The figure shows three views and two pictorial views of one solid part (mm, origin at its lowest corner). Answer the questions. Round coordinates to 2 decimals unless told otherwise and drop trailing zeros. Write each loop counter-clockwise with the first axis right and the second up, starting at its lowest first coordinate (ties: lowest second). Pieces come first, ordered by that corner, then holes. Notation, with made-up numbers: M 10,-19.75 L 63,-19.75 A34 ccw 63,12.25 Z; hole C -12,50.5 d11. An arc over 180 degrees is marked long. One line per item, written item: value. Start each with the question number.
Q1. Find section B-B (x = 10.35). Write down the section's boundary in (y, z) (3 decimals), and give its area (3 significant figures).
Q2. Find section A-A (y = 82.55). Write down the section's boundary in (x, z) (3 decimals), and give its area (3 significant figures).
Q3. Consider probe 1 along X at (y, z) = (82.55, 2.7) (3 decimals); probe 2 along Y at (x, z) = (10.35, 2.9) (3 decimals); probe 3 along Y at (x, z) = (7, 2.7). Determine where each line is inside the solid, lowest interval first.
Q4. Given pin 1 Ø1.2 at (y, z) = (1.5, 2.5) entering from -X; pin 2 Ø2 at (x, z) = (33, 2.5) entering from +Y; pin 3 Ø2 at (x, z) = (23.5, 2.5) entering from -Y, each flat-ended and moving along its own axis, determine where each tip first touches the part or whether it passes through.
Q5. Find section D-D (x = 88). Write down the section's boundary in (y, z), and give its area (3 significant figures).
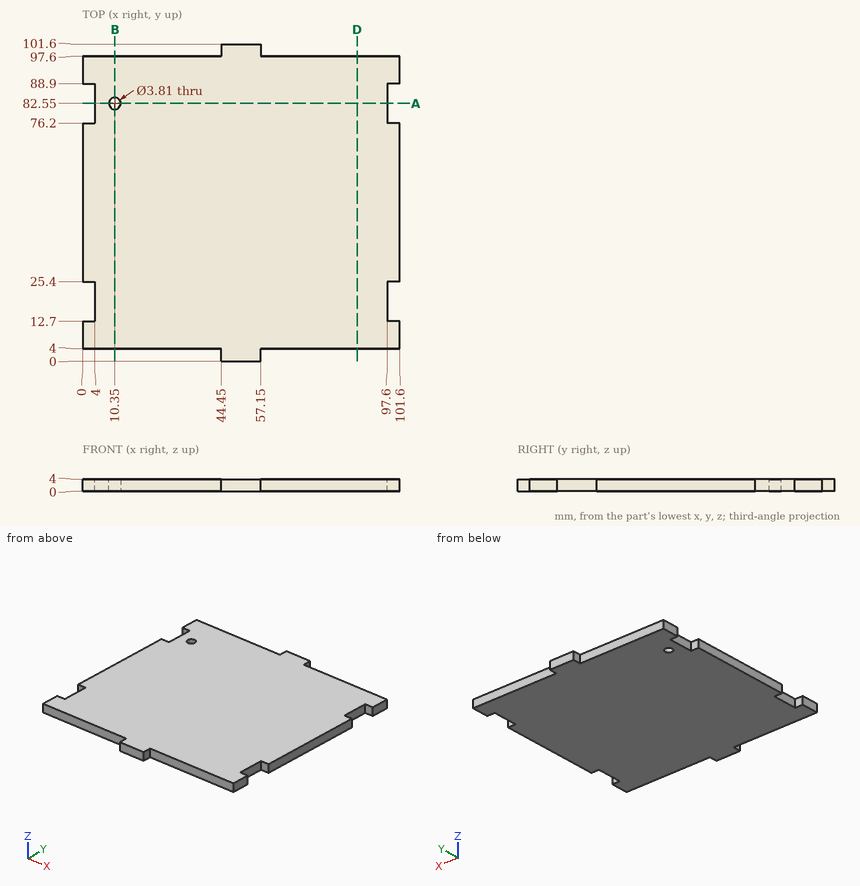
The answers:
1. outline: M 4,0 L 80.645,0 L 80.645,4 L 4,4 Z; M 84.455,0 L 97.6,0 L 97.6,4 L 84.455,4 Z
1. area: 359 mm2
2. outline: M 4,0 L 8.445,0 L 8.445,4 L 4,4 Z; M 12.255,0 L 97.6,0 L 97.6,4 L 12.255,4 Z
2. area: 359 mm2
3. probe 1: 4 to 8.445, 12.255 to 97.6
3. probe 2: 4 to 80.645, 84.455 to 97.6
3. probe 3: 4 to 97.6
4. pin 1: x = 44.45
4. pin 2: y = 97.6
4. pin 3: y = 4
5. outline: M 4,0 L 97.6,0 L 97.6,4 L 4,4 Z
5. area: 374 mm2
